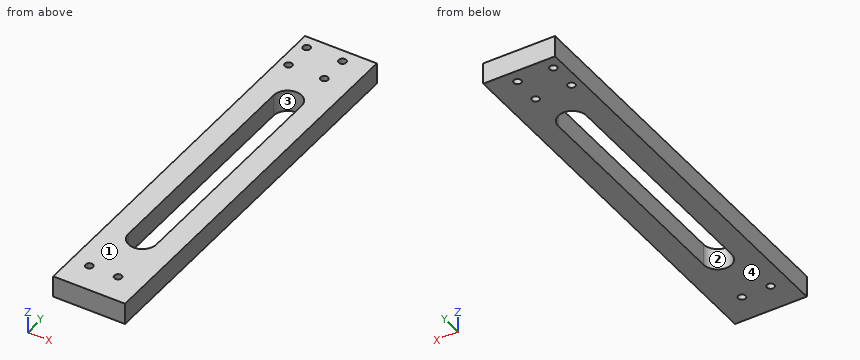
```python
from build123d import *

# Parameters (mm, degrees)
F0_W     = 63.5
F0_H     = 19.05
F1_DEPTH = 176.2125
F3_D     = 6.5278
F5_DEPTH = 19.051


with BuildPart() as f1:
    # F0 (on Front) → F1 (new body, symmetric)
    with BuildSketch(Plane.XZ):
        Rectangle(F0_W, F0_H)
    extrude(amount=F1_DEPTH, both=True)

    # F3 (through all)
    with Locations(Plane.XY.offset(9.525)):
        with Locations((8.7006882876, 164.7427699804), (8.7006882876, 139.3427699804), (-23.0493117124, 139.3427699804), (-23.0493117124, 164.7427699804), (-15.875, -150.8125), (9.525, -150.8125)):
            Hole(F3_D / 2)

    # F4 (on face) → F5 (cut, through all)
    with BuildSketch(Plane.XY.offset(9.525)):
        with BuildLine():
            Line((-12.3660704418, 101.6), (-12.3660704418, -101.6))
            ThreePointArc((-12.3660704418, -101.6), (0, -113.9660704418), (12.3660704418, -101.6))
            Line((12.3660704418, -101.6), (12.3660704418, 101.6))
            ThreePointArc((12.3660704418, 101.6), (0, 113.9660704418), (-12.3660704418, 101.6))
        make_face()
    extrude(amount=-F5_DEPTH, mode=Mode.SUBTRACT)


solid = f1.part
```
The listing builds one solid part. Answer for the finished solid, in the listing's coordinates (mm). Face numbers are marked on the shaded views. A direction names the side the tool comes from. Round coordinates to 2 decimals unless told otherwise and drop trailing zeros. Loops run counter-clockwise (first coordinate to the right, second up) from the corner with the lowest first, then second, coordinate; pieces in that order, holes last. Notation, with made-up numbers: (72, 78.5) - (109, 78.5) arc R21 ccw to (109, 91.5) - close; hole circle Ø7 at (-18, -22). An arc over 180 degrees is marked (long way). Use one line per item in the form item = value. Start each with the question number.
1. The part is cut by section B-B on x = 0. Determine the outline of the cut face in (y, z) (1 decimal).
2. The part is cut by section C-C on z = 1.25. Give the number of separate pieces and of enclosed holes in the cut face, then the cut area to 3 significant figures.
3. Given pin 1 Ø10.5 at (x, y) = (8.7, 139.34) entering from -Z (3 decimals), flat-ended and moving along its own axis, determine where the tip first touches the part or whether it passes through.
4. For a pull along X with two mould halves and no side action, classify the marked faces 1 and 2 as pulls with the +X half, pulls with the -X half, needs draft (parallel to the pull), parting line crosses it, or undercut.
5. The part is cut by section A-A on y = -94.5. Determine the outline of the cut face in (x, z) (3 decimals), then the cut area to 3 significant figures.
6. A tool of negligible diameter and unlimited length cuts with its end or side. For the marked faces 3 and 4, from which of +Z, -Z, +X, -X, +Y, -Y can it reach the whole face along a straight path? Write none if from no direction.
7. Consider line 1 (X direction, y = 25.5, z = -0.75); line 2 (X direction, y = 138, z = 5.5); line 3 (Y direction, x = -17.5, z = 8.5). Determine where each line is inside the solid, lowest interval first. Write a range as [from, to].
Geometry check:
q1.outline = (-176.2, -9.5) - (-114, -9.5) - (-114, 9.5) - (-176.2, 9.5) - close; (114, -9.5) - (176.2, -9.5) - (176.2, 9.5) - (114, 9.5) - close
q2.separate_pieces = 1
q2.enclosed_holes = 7
q2.area = 16,700 mm^2
q3.pin_1 = -9.525
q4.face_1 = needs draft
q4.face_2 = undercut
q5.outline = (-31.75, -9.525) - (-12.366, -9.525) - (-12.366, 9.525) - (-31.75, 9.525) - close; (12.366, -9.525) - (31.75, -9.525) - (31.75, 9.525) - (12.366, 9.525) - close
q5.area = 739 mm^2
q6.face_3 = +Z, -Z
q6.face_4 = -Z, +X, -X, +Y, -Y
q7.line_1 = [-31.75, -12.37], [12.37, 31.75]
q7.line_2 = [-31.75, -26.02], [-20.07, 5.73], [11.68, 31.75]
q7.line_3 = [-176.21, -153.64], [-147.98, 176.21]
